from build123d import *

# Parameters (mm, degrees)
SKETCH1_W           = 200
SKETCH1_H           = 115
SKETCH1_R           = 20
BOSS_EXTRUDE1_DEPTH = 5
CUT_EXTRUDE1_REACH  = 117.461
SKETCH4_R           = 2
SKETCH5_R           = 4
CUT_EXTRUDE2_DEPTH  = 2
FILLET1_R           = 30
SKETCH8_R           = 2
CUT_EXTRUDE4_DEPTH  = 116.461032388
SKETCH11_W          = 71.5
SKETCH11_H          = 71.5
CUT_EXTRUDE7_DEPTH  = 0.5
SKETCH9_W           = 4
SKETCH9_H           = 40.75
CUT_EXTRUDE5_DEPTH  = 116.461032388
CUT_EXTRUDE8_DEPTH  = 2


with BuildPart() as part:
    # Sketch1 → Boss-Extrude1 (new body)
    with BuildSketch(Plane(origin=(0, 0, 0), x_dir=(0, 1, 0), z_dir=(0, 0, 1))):
        Rectangle(SKETCH1_W, SKETCH1_H)
        with Locations(Location((0, 0, 0), (0, 0, 270))):
            Circle(SKETCH1_R, mode=Mode.SUBTRACT)
    extrude(amount=BOSS_EXTRUDE1_DEPTH)

    # Sketch4 → Cut-Extrude1 (cut, up to next)
    with BuildSketch(Plane.XY.offset(5), mode=Mode.PRIVATE) as cut_extrude1_sk1:
        with Locations((29, 29)):
            Circle(SKETCH4_R)
    cut_extrude1_tool1 = extrude(cut_extrude1_sk1.sketch, amount=-CUT_EXTRUDE1_REACH, mode=Mode.PRIVATE) & part.part
    # Sketch4 → Cut-Extrude1 (cut, up to next)
    with BuildSketch(Plane.XY.offset(5), mode=Mode.PRIVATE) as cut_extrude1_sk2:
        with Locations((-29, 29)):
            Circle(SKETCH4_R)
    cut_extrude1_tool2 = extrude(cut_extrude1_sk2.sketch, amount=-CUT_EXTRUDE1_REACH, mode=Mode.PRIVATE) & part.part
    # Sketch4 → Cut-Extrude1 (cut, up to next)
    with BuildSketch(Plane.XY.offset(5), mode=Mode.PRIVATE) as cut_extrude1_sk3:
        with Locations((-29, -29)):
            Circle(SKETCH4_R)
    cut_extrude1_tool3 = extrude(cut_extrude1_sk3.sketch, amount=-CUT_EXTRUDE1_REACH, mode=Mode.PRIVATE) & part.part
    # Sketch4 → Cut-Extrude1 (cut, up to next)
    with BuildSketch(Plane.XY.offset(5), mode=Mode.PRIVATE) as cut_extrude1_sk4:
        with Locations((29, -29)):
            Circle(SKETCH4_R)
    cut_extrude1_tool4 = extrude(cut_extrude1_sk4.sketch, amount=-CUT_EXTRUDE1_REACH, mode=Mode.PRIVATE) & part.part
    add(cut_extrude1_tool1.solids().sort_by_distance((29, 29, 5))[0], mode=Mode.SUBTRACT)
    add(cut_extrude1_tool2.solids().sort_by_distance((-29, 29, 5))[0], mode=Mode.SUBTRACT)
    add(cut_extrude1_tool3.solids().sort_by_distance((-29, -29, 5))[0], mode=Mode.SUBTRACT)
    add(cut_extrude1_tool4.solids().sort_by_distance((29, -29, 5))[0], mode=Mode.SUBTRACT)

    # Sketch5 → Cut-Extrude2 (cut)
    with BuildSketch(Plane.XY.offset(5)):
        with Locations((-29, -29)):
            Circle(SKETCH5_R)
        with Locations((-29, 29)):
            Circle(SKETCH5_R)
        with Locations((29, -29)):
            Circle(SKETCH5_R)
        with Locations((29, 29)):
            Circle(SKETCH5_R)
    extrude(amount=-CUT_EXTRUDE2_DEPTH, mode=Mode.SUBTRACT)

    # Fillet1
    fillet1_edges = [part.edges().sort_by_distance(p)[0] for p in [
        (57.5, 100, 2.5),
        (57.5, -100, 2.5),
        (-57.5, -100, 2.5),
        (-57.5, 100, 2.5),
    ]]
    fillet(fillet1_edges, radius=FILLET1_R)

    # Sketch8 → Cut-Extrude4 (cut, through all)
    with BuildSketch(Plane.XY.offset(5)):
        with Locations((15, 88.5)):
            Circle(SKETCH8_R)
        with Locations((-15, 88.5)):
            Circle(SKETCH8_R)
        with Locations((-14.960853972, -88.5)):
            Circle(SKETCH8_R)
        with Locations((15.039146028, -88.5)):
            Circle(SKETCH8_R)
    extrude(amount=-CUT_EXTRUDE4_DEPTH, mode=Mode.SUBTRACT)

    # Sketch11 → Cut-Extrude7 (cut)
    with BuildSketch(Plane(origin=(0, 0, 0), x_dir=(1, 0, 0), z_dir=(0, 0, -1))):
        Rectangle(SKETCH11_W, SKETCH11_H)
    extrude(amount=-CUT_EXTRUDE7_DEPTH, mode=Mode.SUBTRACT)

    # Sketch9 → Cut-Extrude5 (cut, through all)
    with BuildSketch(Plane.XY.offset(5)):
        with Locations((30.875, 61.125)):
            Rectangle(SKETCH9_W, SKETCH9_H)
        with Locations((-30.875, 61.125)):
            Rectangle(SKETCH9_W, SKETCH9_H)
    extrude(amount=-CUT_EXTRUDE5_DEPTH, mode=Mode.SUBTRACT)

    # Sketch12 → Cut-Extrude8 (cut)
    with BuildSketch(Plane(origin=(0, 0, 0), x_dir=(1, 0, 0), z_dir=(0, 0, -1))):
        with BuildLine():
            Line((-34.125, -81.5), (-34.125, -40.75))
            ThreePointArc((-34.125, -40.75), (-30.875, -37.5), (-27.625, -40.75))
            Line((-27.625, -40.75), (-27.625, -81.5))
            ThreePointArc((-27.625, -81.5), (-30.875, -84.75), (-34.125, -81.5))
        make_face()
        with BuildLine():
            Line((34.125, -81.5), (34.125, -40.75))
            ThreePointArc((34.125, -40.75), (30.875, -37.5), (27.625, -40.75))
            Line((27.625, -40.75), (27.625, -81.5))
            ThreePointArc((27.625, -81.5), (30.875, -84.75), (34.125, -81.5))
        make_face()
    extrude(amount=-CUT_EXTRUDE8_DEPTH, mode=Mode.SUBTRACT)


solid = part.part
Input: part model. Units: mm. Frame: model coordinates. A direction names the side the tool comes from. Round coordinates to 2 decimals unless told otherwise and drop trailing zeros. Order: outer loops, then holes, each group sorted by start corner. A loop starts at its lowest first (then second) coordinate and runs counter-clockwise, first axis right, second up. Notation, with made-up numbers: (-31, 32) - (-24, 32) arc R17 cw to (-24, 50) - close; hole circle Ø1 at (3, -17.75). An arc over 180 degrees is marked (long way). Use a Markdown table: item, result.
1. Section B-B on x = 0. Return the cut outline in (y, z).
Evaluation:
| item | result |
|---|---|
| outline | (-100, 0) - (-35.75, 0) - (-35.75, 0.5) - (-20, 0.5) - (-20, 5) - (-100, 5) - close; (20, 0.5) - (35.75, 0.5) - (35.75, 0) - (100, 0) - (100, 5) - (20, 5) - close |
2. Access query for faces 1 (the face through (30, -27, 3)), 2 (the face through (-16, -16, 0.5)), 3 (the face through (0, -100, 2)). Directions: +Z, -Z, +X, -X, +Y, -Y. A direction counts if a zero-diameter tool reaches every point of the face in a straight line with its end or side. Return the directions, or none.
Evaluation:
| item | result |
|---|---|
| face 1 | +Z |
| face 2 | -Z |
| face 3 | +Z, -Z, +X, -X, -Y |
3. Material intervals for probe 1 along Y at (x, z) = (29, 4.1); probe 2 along X at (y, z) = (62, 4.65) (3 decimals); probe 3 along Y at (x, z) = (-10.5, 1.9), sorted ascending.
Evaluation:
| item | result |
|---|---|
| probe 1 | -99.96 to -33, -25 to 25, 33 to 40.75, 81.5 to 99.96 |
| probe 2 | -57.5 to -32.875, -28.875 to 28.875, 32.875 to 57.5 |
| probe 3 | -100 to -17.02, 17.02 to 100 |
4. First-contact query: pin 1 (2.5 mm diameter, centred on x = 30.5, z = 3, fed in from -Y). Flat tip, straight axial feed; report the tip coordinate or a pass-through.
Evaluation:
| item | result |
|---|---|
| pin 1 | y = -99.95 |
5. Mould query, pull axis X, two halves, no side actions, for faces 4 (the face through (48.945, 90.979, 2.535)), 5 (the face through (-48.945, 90.979, 2.535)), 6 (the face through (28.479, -25.034, 4.014)), 7 (the face through (38, -1, 0)). Classes: +X half, -X half, draft (parallel to the pull), parting line (faces both ways), or undercut.
Evaluation:
| item | result |
|---|---|
| face 4 | +X half |
| face 5 | -X half |
| face 6 | undercut |
| face 7 | draft |
6. Section C-C on x = 22. Return the cut outline in (y, z), then the cut area to 3 significant figures.
Evaluation:
| item | result |
|---|---|
| outline | (-100, 0) - (-35.75, 0) - (-35.75, 0.5) - (35.75, 0.5) - (35.75, 0) - (100, 0) - (100, 5) - (-100, 5) - close |
| area | 964 mm^2 |
7. Section D-D on x = -15. Return the cut outline in (y, z), then the cut area to 3 significant figures.
Evaluation:
| item | result |
|---|---|
| outline | (-100, 0) - (-90.5, 0) - (-90.5, 5) - (-100, 5) - close; (-86.5, 0) - (-35.75, 0) - (-35.75, 0.5) - (-13.23, 0.5) - (-13.23, 5) - (-86.5, 5) - close; (13.23, 0.5) - (35.75, 0.5) - (35.75, 0) - (86.5, 0) - (86.5, 5) - (13.23, 5) - close; (90.5, 0) - (100, 0) - (100, 5) - (90.5, 5) - close |
| area | 805 mm^2 |
8. Section A-A on y = -29. Return the cut outline in (x, z), then the cut area to 3 significant figures.
Evaluation:
| item | result |
|---|---|
| outline | (-57.5, 0) - (-35.75, 0) - (-35.75, 0.5) - (-31, 0.5) - (-31, 3) - (-33, 3) - (-33, 5) - (-57.5, 5) - close; (-27, 0.5) - (27, 0.5) - (27, 3) - (25, 3) - (25, 5) - (-25, 5) - (-25, 3) - (-27, 3) - close; (31, 0.5) - (35.75, 0.5) - (35.75, 0) - (57.5, 0) - (57.5, 5) - (33, 5) - (33, 3) - (31, 3) - close |
| area | 487 mm^2 |
